The figure shows three views and two pictorial views of one solid part (mm, origin at its lowest corner). Answer the questions. A direction names the side the tool comes from. Give positions to 0.01 mm unless a question says otherwise; leave off trailing zeros. Loops run counter-clockwise (first coordinate to the right, second up) from the corner with the lowest first, then second, coordinate; pieces in that order, holes last. Notation, with made-up numbers: (34, 15.25) - (85, 15.25) arc R19 cw to (85, 23.25) - close; hole circle Ø7 at (41.25, -3). An arc over 180 degrees is marked (long way). Use a Markdown table: item, result. Add a question column.
Item 1: Which of the six approach directions +Z, -Z, +X, -X, +Y, -Y give full straight-line access (tool end or side, diameter ignored) to the marked faces 3 and 4?
Item 2: Consider probe 1 along Y at (x, z) = (3.5, 5.5); probe 2 along Z at (x, y) = (1.75, 5.5); probe 3 along X at (y, z) = (2.5, 6.5). Determine where each line is inside the solid, lowest interval first. Write a range as [from, to].
Item 3: A cutting plane is placed at D-D (z = 2.75). Determine the outline of the cut face in (x, y), plus the area to 3 significant figures.
Item 4: A cutting plane is placed at C-C (x = 2.75). Determine the outline of the cut face in (y, z).
Item 5: A cutting plane is placed at B-B (y = 2.75). Determine the outline of the cut face in (x, z).
Item 6: For a pull along X with two mould halves and no side action, classify the marked faces 1 and 2 as +X half, -X half, draft (parallel to the pull), parting line (faces both ways), or undercut.
Item 7: A cutting plane is placed at A-A (z = 8.5). Determine the outline of the cut face in (x, y), plus the area to 3 significant figures.
Item 8: Each of these flat-tipped pins is pushed along its axis until it touches: P1, Ø1, axis at y = 4.5, z = 4, coming from the -X side; P2, Ø2, axis at x = 4, z = 6, coming from the +Y side; P3, Ø2, axis at y = 4.5, z = 3, coming from the -X side. Where does it stop, or does it pass through?
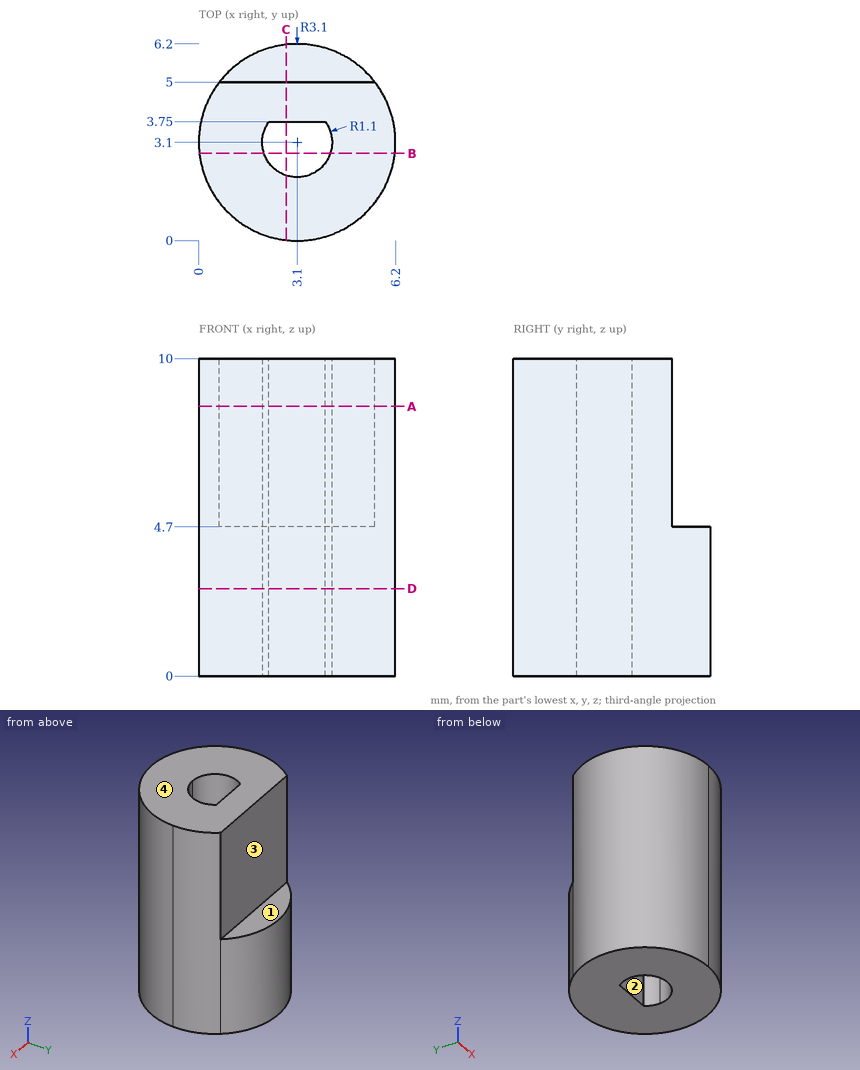
Geometry says:
| question | item | result |
|---|---|---|
| 1 | face 3 | +Z, +X, -X, +Y |
| 1 | face 4 | +Z, +X, -X, +Y, -Y |
| 2 | probe 1 | [0.03, 2.08], [3.75, 5] |
| 2 | probe 2 | [0, 4.7] |
| 2 | probe 3 | [0.06, 2.18], [4.02, 6.14] |
| 3 | outline | circle Ø6.2 at (3.1, 3.1); hole (2.21, 3.75) arc R1.1 ccw (long way) to (3.99, 3.75) - close |
| 3 | area | 26.9 mm² |
| 4 | outline | (0.02, 0) - (2.06, 0) - (2.06, 10) - (0.02, 10) - close; (3.75, 0) - (6.18, 0) - (6.18, 4.7) - (5, 4.7) - (5, 10) - (3.75, 10) - close |
| 5 | outline | (0.02, 0) - (2.06, 0) - (2.06, 10) - (0.02, 10) - close; (4.14, 0) - (6.18, 0) - (6.18, 10) - (4.14, 10) - close |
| 6 | face 1 | draft |
| 6 | face 2 | undercut |
| 7 | outline | (0.65, 5) arc R3.1 ccw (long way) to (5.55, 5) - close; hole (2.21, 3.75) arc R1.1 ccw (long way) to (3.99, 3.75) - close |
| 7 | area | 22.8 mm² |
| 8 | P1 | x = 0.13 |
| 8 | P2 | y = 5 |
| 8 | P3 | x = 0.03 |
